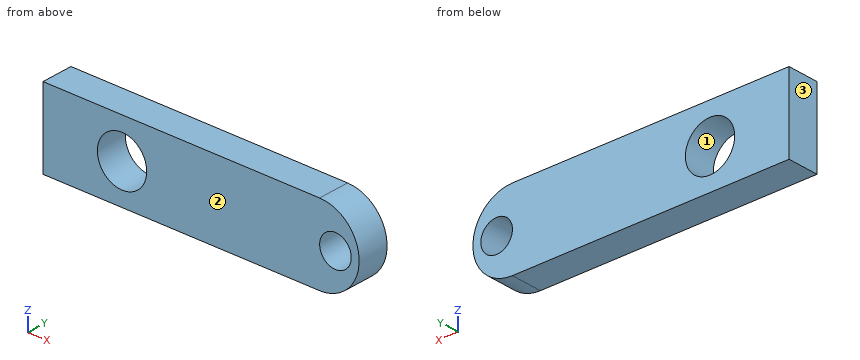
Autodesk Inventor part; units mm, degrees
ref_plane "YZ Plane" through (0, 0, 0) normal (1, 0, 0) x (0, 1, 0)
ref_plane "XZ Plane" through (0, 0, 0) normal (0, 1, 0) x (-1, 0, 0)
ref_plane "XY Plane" through (0, 0, 0) normal (0, 0, 1) x (1, 0, 0)
sketch "Sketch1" plane through (0, 0, 0) normal (0, 1, 0) x (-1, 0, 0)
  line L0 (0, 0) -> (87.5, 0)
  line L1 (87.5, 0) -> (87.5, 25)
  line L2 (87.5, 25) -> (0, 25)
  circle A0 centre (62.5, 12.5) radius 7.8
  arc A1 (0, 25) -> (0, 0) centre (0, 12.5) ccw
  circle A2 centre (-5, 12.5) radius 5
extrude "Extrusion1" add sketch "Sketch1" along normal blind 10
properties part number "handle_crank" material "Plywood, Finish"
Verification items for the finished model (mm, model axes). Face numbers are marked on the shaded views. Coordinates: 2 decimals unless noted, no trailing zeros. Loops run counter-clockwise (first coordinate to the right, second up) from the corner with the lowest first, then second, coordinate; pieces in that order, holes last. Notation, with made-up numbers: (-20, 59.25) -> (10, 59.25) arc R26 cw to (10, 93.25) -> close; hole circle Ø6 at (37, -36). An arc over 180 degrees is marked (long way). Answer in a Markdown table with one row per item. Add a question column.
1. Section check D-D, the plane z = 18.5. Enter the section's corners in (x, y).
2. Material ranges on probe 1 along Z at (x, y) = (-62.5, 5.5); probe 2 along X at (y, z) = (8, 9.25); probe 3 along X at (y, z) = (6.75, 13.5), recorded low to high. Write a range as [from, to].
3. Section check A-A, the plane x = -62.5. Enter the section's corners in (y, z), then the cut area to 3 significant figures.
4. Section check C-C, the plane y = 7. Enter the section's corners in (x, z).
5. Depth check by flat-ended pin: P1, Ø12.5, axis at x = -62.5, z = 12.5, coming from the +Y side; P2, Ø6, axis at y = 3.5, z = 20.5, coming from the +X side; P3, Ø6, axis at y = 4, z = 4, coming from the +X side (3 decimals). Enter the tip coordinate at first touch or a pass-through.
6. Section check B-B, the plane z = 8.5. Enter the section's corners in (x, y).
7. Draft check along X on the marked faces 1, 2 and 3. Enter one of: +X half, -X half, draft (parallel to the pull), parting line (faces both ways), or undercut.
Derived:
| question | item | result |
|---|---|---|
| 1 | outline | (-87.5, 0) -> (-67.48, 0) -> (-67.48, 10) -> (-87.5, 10) -> close; (-57.52, 0) -> (10.97, 0) -> (10.97, 10) -> (-57.52, 10) -> close |
| 2 | probe 1 | z = [0, 4.7], [20.3, 25] |
| 2 | probe 2 | x = [-87.5, -69.59], [-55.41, 1.2], [8.8, 12.07] |
| 2 | probe 3 | x = [-87.5, -70.24], [-54.76, 0.1], [9.9, 12.46] |
| 3 | outline | (0, 0) -> (10, 0) -> (10, 4.7) -> (0, 4.7) -> close; (0, 20.3) -> (10, 20.3) -> (10, 25) -> (0, 25) -> close |
| 3 | area | 94.0 mm² |
| 4 | outline | (-87.5, 0) -> (0, 0) arc R12.5 ccw to (0, 25) -> (-87.5, 25) -> close; hole circle Ø15.6 at (-62.5, 12.5); hole circle Ø10 at (5, 12.5) |
| 5 | P1 | passes through |
| 5 | P2 | stops at x = 11.46 |
| 5 | P3 | stops at x = 11.225 |
| 6 | outline | (-87.5, 0) -> (-69.2, 0) -> (-69.2, 10) -> (-87.5, 10) -> close; (-55.8, 0) -> (2, 0) -> (2, 10) -> (-55.8, 10) -> close; (8, 0) -> (11.84, 0) -> (11.84, 10) -> (8, 10) -> close |
| 7 | face 1 | undercut |
| 7 | face 2 | draft |
| 7 | face 3 | -X half |
